Input: part model. Units: mm. Frame: model coordinates. Give positions to 0.01 mm unless a question says otherwise; leave off trailing zeros. Return JSON: item names as keys, results as strings. Group by question number.
```python
from build123d import *

# Parameters (mm, degrees)
SKETCH_1_W      = 14
SKETCH_1_H      = 14
SKETCH_1_W_2    = 11.6
SKETCH_1_H_2    = 11.6
SKETCH_1_W_3    = 4.6
SKETCH_1_H_3    = 4.6
EXTRUDE_2_DEPTH = 2000


with BuildPart() as part:
    # Эскиз1 → Бобышка-Вытянуть2 (new body)
    # profile 1 of 9: a face of its own
    with BuildSketch(Plane(origin=(0, 0, 0), x_dir=(1, 0, 0), z_dir=(0, 1, 0))):
        Polygon((8, -7), (8, -6.151471863), (6, -8.151471863), (6, -13.6), (-6, -13.6), (-6, -8.151471863), (-8, -6.151471863), (-8, -7), (-8.848528137, -7), (-7, -8.848528137), (-7, -13.4), (-8.9, -13.4), (-8.9, -12.8), (-10.9, -12.8), (-10.9, -14.2), (-10.4, -14.2), (-10.4, -15), (10.4, -15), (10.4, -14.2), (10.9, -14.2), (10.9, -12.8), (8.9, -12.8), (8.9, -13.4), (7, -13.4), (7, -8.848528137), (8.848528137, -7), align=None)
    # profile 2 of 9: a face of its own
    with BuildSketch(Plane(origin=(0, 0, 0), x_dir=(1, 0, 0), z_dir=(0, 1, 0))):
        with Locations((-15, 0)):
            Rectangle(SKETCH_1_W, SKETCH_1_H)
        with Locations((-15, 0)):
            Rectangle(SKETCH_1_W_2, SKETCH_1_H_2, mode=Mode.SUBTRACT)
    # profile 3 of 9: a face of its own
    with BuildSketch(Plane(origin=(0, 0, 0), x_dir=(1, 0, 0), z_dir=(0, 1, 0))):
        Polygon((-23, -8.848528137), (-21.151471863, -7), (-22, -7), (-22, -6.151471863), (-23.848528137, -8), (-28.4, -8), (-28.4, -6.1), (-27.8, -6.1), (-27.8, -4.1), (-29.2, -4.1), (-29.2, -4.6), (-30, -4.6), (-30, -15), (-19.6, -15), (-19.6, -14.2), (-19.1, -14.2), (-19.1, -12.8), (-21.1, -12.8), (-21.1, -13.4), (-23, -13.4), align=None)
        with Locations((-26.3, -11.3)):
            Rectangle(SKETCH_1_W_3, SKETCH_1_H_3, mode=Mode.SUBTRACT)
    # profile 4 of 9: a face of its own
    with BuildSketch(Plane(origin=(0, 0, 0), x_dir=(1, 0, 0), z_dir=(0, 1, 0))):
        with Locations((15, 0)):
            Rectangle(SKETCH_1_W, SKETCH_1_H)
        with Locations((15, 0)):
            Rectangle(SKETCH_1_W_2, SKETCH_1_H_2, mode=Mode.SUBTRACT)
    # profile 5 of 9: a face of its own
    with BuildSketch(Plane(origin=(0, 0, 0), x_dir=(1, 0, 0), z_dir=(0, 1, 0))):
        Polygon((23.848528137, -8), (22, -6.151471863), (22, -7), (21.151471863, -7), (23, -8.848528137), (23, -13.4), (21.1, -13.4), (21.1, -12.8), (19.1, -12.8), (19.1, -14.2), (19.6, -14.2), (19.6, -15), (30, -15), (30, -4.6), (29.2, -4.6), (29.2, -4.1), (27.8, -4.1), (27.8, -6.1), (28.4, -6.1), (28.4, -8), align=None)
        with Locations((26.3, -11.3)):
            Rectangle(SKETCH_1_W_3, SKETCH_1_H_3, mode=Mode.SUBTRACT)
    # profile 6 of 9: a face of its own
    with BuildSketch(Plane(origin=(0, 0, 0), x_dir=(1, 0, 0), z_dir=(0, 1, 0))):
        Polygon((21.151471863, 7), (22, 7), (22, 6.151471863), (23.848528137, 8), (28.4, 8), (28.4, 6.1), (27.8, 6.1), (27.8, 4.1), (29.2, 4.1), (29.2, 4.6), (30, 4.6), (30, 15), (19.6, 15), (19.6, 14.2), (19.1, 14.2), (19.1, 12.8), (21.1, 12.8), (21.1, 13.4), (23, 13.4), (23, 8.848528137), align=None)
        with Locations((26.3, 11.3)):
            Rectangle(SKETCH_1_W_3, SKETCH_1_H_3, mode=Mode.SUBTRACT)
    # profile 7 of 9: a face of its own
    with BuildSketch(Plane(origin=(0, 0, 0), x_dir=(1, 0, 0), z_dir=(0, 1, 0))):
        Polygon((8, 7), (8.848528137, 7), (7, 8.848528137), (7, 13.4), (8.9, 13.4), (8.9, 12.8), (10.9, 12.8), (10.9, 14.2), (10.4, 14.2), (10.4, 15), (-10.4, 15), (-10.4, 14.2), (-10.9, 14.2), (-10.9, 12.8), (-8.9, 12.8), (-8.9, 13.4), (-7, 13.4), (-7, 8.848528137), (-8.848528137, 7), (-8, 7), (-8, 6.151471863), (-6, 8.151471863), (-6, 13.6), (6, 13.6), (6, 8.151471863), (8, 6.151471863), align=None)
    # profile 8 of 9: a face of its own
    with BuildSketch(Plane(origin=(0, 0, 0), x_dir=(1, 0, 0), z_dir=(0, 1, 0))):
        Polygon((-22, 7), (-21.151471863, 7), (-23, 8.848528137), (-23, 13.4), (-21.1, 13.4), (-21.1, 12.8), (-19.1, 12.8), (-19.1, 14.2), (-19.6, 14.2), (-19.6, 15), (-30, 15), (-30, 13.6), (-28.6, 13.6), (-24, 13.6), (-24, 9), (-24, 8.151471863), (-23.848528137, 8), (-22, 6.151471863), align=None)
    # profile 9 of 9: a face of its own
    with BuildSketch(Plane(origin=(0, 0, 0), x_dir=(1, 0, 0), z_dir=(0, 1, 0))):
        Polygon((-28.6, 13.6), (-30, 13.6), (-30, 4.6), (-29.2, 4.6), (-29.2, 4.1), (-27.8, 4.1), (-27.8, 6.1), (-28.4, 6.1), (-28.4, 8), (-23.848528137, 8), (-24, 8.151471863), (-24, 9), (-28.6, 9), align=None)
    extrude(amount=EXTRUDE_2_DEPTH)


solid = part.part
```
Item 1: Section A-A, the plane y = 1661.5. Give the number of separate pieces and of enclosed holes in the cut face, then the cut area to 3 significant figures.
Item 2: Material intervals for line 1 (Z direction, x = 25.5, y = 262); line 2 (X direction, y = 701, z = 3.25); line 3 (X direction, y = 299, z = -5), sorted ascending. Write a range as from..to.
Item 3: First-contact query: pin 1 Ø2 at (y, z) = (775.5, -1.5) entering from +X; pin 2 Ø4 at (x, z) = (17, 11) entering from +Y. Flat tips, straight axial feed; report the tip coordinate or a pass-through.
Answer below:
{
 "1": {"separate pieces": "1", "enclosed holes": "7", "area": "400 mm^2"},
 "2": {"line 1": "-15..-13.6, -9..-8, 8..9, 13.6..15", "line 2": "-22..-20.8, -9.2..-8, 8..9.2, 20.8..22", "line 3": "-30..-27.8, -22..-20.8, -9.2..-8, 8..9.2, 20.8..22, 27.8..30"},
 "3": {"pin 1": "x = 22", "pin 2": "through"}
}
